Build history of the part. All positions in model axes, mm. Face numbers are marked on the shaded views. A direction names the side the tool comes from. Give positions to 0.01 mm unless a question says otherwise; leave off trailing zeros. Loops run counter-clockwise (first coordinate to the right, second up) from the corner with the lowest first, then second, coordinate; pieces in that order, holes last.
1) Band-saw the part on B-B on y = 0.75. List the corners of the cut face in (x, z), then the cut area to 3 significant figures.
2) Two-plate mould, pull along X, no slides. Class the marked faces 6, 7 and 8: +X half, -X half, draft (parallel to the pull), parting line (faces both ways), or undercut.
3) Band-saw the part on D-D on x = 19.5. List the corners of the cut face in (y, z), then the cut area to 3 significant figures.
4) Wall check: line 1 (Y direction, x = 0, z = 3.75) (3 decimals); line 2 (X direction, y = 14.75, z = 5.75); line 3 (Y direction, x = -19.5, z = 8.5). Give the ranges that are in metal, low to high.
5) 3-axis set-ups, long thin cutter, end or side, ignore diameter. For the marked faces 1, 2, 3, 4 and 5: which of +Z, -Z, +X, -X, +Y, -Y reach the whole face in a straight line?
6) Band-saw the part on A-A on x = 0. List the corners of the cut face in (y, z) (3 decimals).
7) Band-saw the part on C-C on z = 2.5. List the corners of the cut face in (x, y) (3 decimals), then the cut area to 3 significant figures.
8) Flat gauge pins, fed straight in: P1, Ø1.5, axis at x = -16.5, y = 13.5, coming from the -Z side; P2, Ø0.8, axis at x = 4.5, z = 5, coming from the +Y side; P3, Ø5, axis at x = 20.5, z = 4.5, coming from the +Y side; P4, Ø1.9, axis at x = 6, z = 9, coming from the +Y side. Where does each tip first touch, or does it go through?
Autodesk Inventor part; units mm, degrees
ref_plane "YZ Plane" through (0, 0, 0) normal (1, 0, 0) x (0, 1, 0)
ref_plane "XZ Plane" through (0, 0, 0) normal (0, 1, 0) x (-1, 0, 0)
ref_plane "XY Plane" through (0, 0, 0) normal (0, 0, 1) x (1, 0, 0)
sketch "Sketch1" plane through (0, 0, 0) normal (0, 0, 1) x (1, 0, 0)
  circle A0 centre (0, 0.75) radius 6.45
  circle A1 centre (0, -8.775) radius 1.9
  line L0 (-18.9, 0) -> (18.9, 0) construction
  line L1 (0, -17.6918) -> (0, 22.1508) construction
  line L2 (-0.5, 16.459) -> (-0.5, 8.23)
  line L3 (-0.5, 8.23) -> (0.5, 8.23)
  line L4 (0.5, 8.23) -> (0.5, 16.4588)
  line L5 (-12.7, 16.459) -> (-0.5, 16.459)
  line L6 (0.5, 16.4588) -> (12.7, 16.4588)
  line L7 (-12.7, 16.459) -> (-13.5, 16.459)
  line L8 (12.7, 16.4588) -> (13.5, 16.4588)
  line L9 (13.5, 16.4588) -> (13.5, 0)
  line L10 (-13.5, 16.459) -> (-13.5, 0)
  arc A2 (-13.5, 0) -> (13.5, 0) centre (0, 1.5937) ccw
  dimension "d0" = 12.9
  dimension "d1" = 3.8
  dimension "d11" = 1
  dimension "d33" = 0.8
  dimension "d34" = 0.8
  dimension "d35" = 27
  dimension "d36" = 13
  dimension "d37" = 13.5
  dimension "d40" = 15.709
  dimension "d44" = 13.5938
  dimension "d45" = 9.525
  dimension "d47" = 15.7088
  dimension "d54" = 7.48
  dimension "d55" = 6.6363
extrude "Extrusion1" add sketch "Sketch1" along normal blind 10
sketch "Sketch2" plane through (0.5, 16.4588, 0) normal (0, 1, 0) x (1, 0, 0)
  line L0 (0, 0) -> (0, -10)
  line L1 (0, -10) -> (7.63, -10)
  line L2 (7.63, -10) -> (7.63, -6.2)
  line L3 (7.63, -6.2) -> (0, -6.2)
  line L4 (0, -6.2) -> (0, -10)
  line L5 (-1, -10) -> (-14, -10)
  line L6 (-1, -10) -> (-8.63, -10)
  line L7 (-8.63, -10) -> (-8.63, -6.2)
  line L8 (-8.63, -6.2) -> (-1, -6.2)
  line L9 (-1, -6.2) -> (-1, -10)
  line L10 (-8.63, -6.2) -> (7.63, -6.2)
  line L11 (7.63, -6.2) -> (7.63, -4.5)
  line L12 (7.63, -4.5) -> (-8.63, -4.5)
  line L13 (-8.63, -4.5) -> (-8.63, -6.2)
  point P0 (-0.5, 0)
  point P1 (-13.2, -10)
  point P2 (7.63, -6.2)
  point P3 (-8.63, -10)
  dimension "d18" = 7.63
  dimension "d19" = 3.8
  dimension "d20" = 7.63
  dimension "d21" = 3.8
  dimension "d22" = 1.7
extrude "Extrusion2" cut sketch "Sketch2" against normal blind 8 contours L10 L8 L13 L12 L0 | L0 L12 L11 L3
extrude "Extrusion3" cut sketch "Sketch2" against normal blind 0.85 contours L3 L2 L1 L0 | L9 L5 L7 L8
sketch "Sketch4" plane through (13.5, 0, 0) normal (1, 0, 0) x (0, 0, -1)
  line L0 (0, 0) -> (-10, 0)
  line L1 (0, 0) -> (0, 16.4588)
  line L2 (-10, 0) -> (0, 0)
  line L3 (0, 0) -> (0, 6)
  line L4 (0, 6) -> (-10, 6)
  line L5 (-10, 6) -> (-10, 0)
  dimension "d56" = 6
extrude "Extrusion5" add sketch "Sketch4" along normal blind 11.11
sketch "Sketch5" plane through (-13.5, 16.459, 0) normal (0, 1, 0) x (1, 0, 0)
  point P0 (13.5, 0)
sketch "Sketch6" plane through (-13.5, 16.459, 0) normal (0, 1, 0) x (1, 0, 0)
  line L0 (5.37, -6.2) -> (5.37, -4.5)
  line L1 (13, 0) -> (13, -10)
  line L2 (5.37, -6.2) -> (13, -6.2)
  line L3 (13, -6.2) -> (13, -10)
  line L4 (13, -10) -> (5.37, -10)
  line L5 (5.37, -10) -> (5.37, -6.2)
  line L6 (5.37, -4.5) -> (13, -4.5)
  line L7 (5.37, -6.2) -> (13, -6.2)
  line L8 (13, -6.2) -> (13, -4.5)
  line L9 (13, -4.5) -> (5.37, -4.5)
  line L10 (5.37, -4.5) -> (5.37, -6.2)
  point P0 (13.5, 0)
extrude "Extrusion6" cut sketch "Sketch6" against normal up to surface (0.8502 mm away) contours L2 L1 L4 L5
extrude "Extrusion7" cut sketch "Sketch6" against normal blind 8 contours L0 L6 L1 L2
sketch "Sketch7" plane through (-13.5, 0, 0) normal (-1, 0, 0) x (0, 0, 1)
  line L0 (0, 16.459) -> (10, 16.459)
  line L1 (10, 16.459) -> (10, 0)
  line L2 (0, 16.459) -> (10, 16.459)
  line L3 (10, 16.459) -> (10, 9.159)
  line L4 (10, 9.159) -> (0, 9.159)
  line L5 (0, 9.159) -> (0, 16.459)
  point P0 (0, 0)
  dimension "d63" = 7.3
extrude "Extrusion8" add sketch "Sketch7" along normal blind 14
sketch "Sketch8" plane through (-13.5, 9.159, 0) normal (0, -1, 0) x (1, 0, 0)
  line L0 (13, 0) -> (-14, 0)
  line L1 (27, 10) -> (0, 10)
  line L2 (-14, 0) -> (0, 0)
  line L3 (0, 0) -> (0, 10)
  line L4 (0, 10) -> (-14, 10)
  line L5 (-14, 10) -> (-14, 0)
  point P0 (13.5, 0)
extrude "Extrusion9" add sketch "Sketch8" along normal blind 7
move faces "Move1" translate (-1, 0, 0) faces at (-27.5, 11.6923, 6.6667)
properties part number "Prowadnica_tloka" material "PC/ABS Plastic"
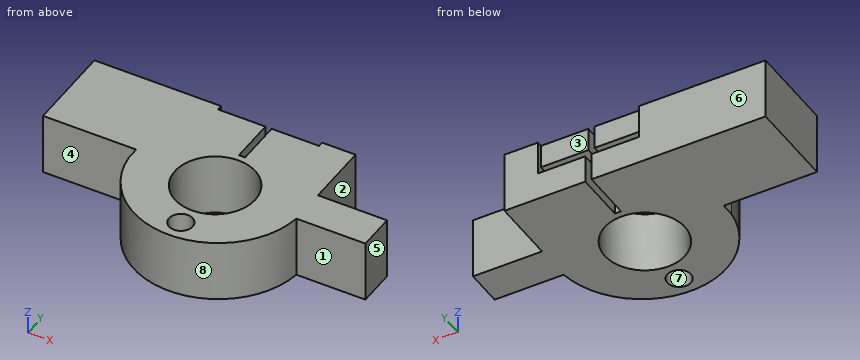
Findings below:
1. outline: (-13.5, 0) - (-6.45, 0) - (-6.45, 10) - (-13.5, 10) - close; (6.45, 0) - (24.61, 0) - (24.61, 10) - (6.45, 10) - close
1. area: 252 mm2
2. face 6: draft
2. face 7: undercut
2. face 8: parting line
3. outline: (0, 0) - (6, 0) - (6, 10) - (0, 10) - close
3. area: 60.0 mm2
4. line 1: y = -12 to -10.675, -6.875 to -5.7, 7.2 to 8.23
4. line 2: x = -28.5 to -8.13, 8.13 to 13.5
4. line 3: y = 2.16 to 16.46
5. face 1: +Z, -Z, +X, -Y
5. face 2: +Z, -Z, +X, +Y
5. face 3: +Z, +Y
5. face 4: +Z, -Z, -X, -Y
5. face 5: +Z, -Z, +X, +Y, -Y
6. outline: (-12, 0) - (-10.675, 0) - (-10.675, 10) - (-12, 10) - close; (-6.875, 0) - (-5.7, 0) - (-5.7, 10) - (-6.875, 10) - close; (7.2, 0) - (8.23, 0) - (8.23, 10) - (7.2, 10) - close
7. outline: (-28.5, 2.159) - (-13.5, 2.159) - (-13.5, 0) arc R13.594 ccw to (13.5, 0) - (24.61, 0) - (24.61, 6) - (13.5, 6) - (13.5, 16.459) - (0.5, 16.459) - (0.5, 8.23) - (-0.5, 8.23) - (-0.5, 16.459) - (-28.5, 16.459) - close; hole circle Ø12.9 at (0, 0.75); hole circle Ø3.8 at (0, -8.775)
7. area: 822 mm2
8. P1: stops at z = 0
8. P2: stops at y = 8.46
8. P3: stops at y = 6
8. P4: stops at y = 15.61
